from build123d import *

# Parameters (mm, degrees)
SKETCH1_W           = 115
SKETCH1_H           = 45
SKETCH1_R           = 6.125
BOSS_EXTRUDE1_DEPTH = 3
SKETCH2_W           = 5
SKETCH2_H           = 45
BOSS_EXTRUDE2_DEPTH = 5
SKETCH3_R           = 1.45
CUT_EXTRUDE1_DEPTH  = 97.276078541
SKETCH4_W           = 5
SKETCH4_H           = 3
BOSS_EXTRUDE3_DEPTH = 122
BOSS_EXTRUDE5_DEPTH = 3
SKETCH8_W           = 5
SKETCH8_H           = 3
BOSS_EXTRUDE6_DEPTH = 12
SKETCH9_W           = 5
SKETCH9_H           = 3
BOSS_EXTRUDE7_DEPTH = 12
SKETCH10_W          = 5
SKETCH10_H          = 3
SKETCH10_H_2        = 5
BOSS_EXTRUDE8_DEPTH = 41.999995
SKETCH13_R          = 1.5
CUT_EXTRUDE3_DEPTH  = 160.289306921


with BuildPart() as part:
    # Sketch1 → Boss-Extrude1 (new body)
    with BuildSketch(Plane.XY):
        with Locations((-27.46518875, -74.528475384)):
            Rectangle(SKETCH1_W, SKETCH1_H)
        Polygon((-16.746917184, -94.028475384), (-38.183460316, -94.028475384), (-27.46518875, -77.307971742), align=None, mode=Mode.SUBTRACT)
        Polygon((-14.96518875, -57.807971742), (-14.96518875, -91.248979027), (-25.683460316, -74.528475384), align=None, mode=Mode.SUBTRACT)
        Polygon((-38.183460316, -55.028475384), (-16.746917184, -55.028475384), (-27.46518875, -71.748979027), align=None, mode=Mode.SUBTRACT)
        Polygon((-39.96518875, -91.248979027), (-39.96518875, -57.807971742), (-29.246917184, -74.528475384), align=None, mode=Mode.SUBTRACT)
        with BuildLine():
            Line((-11.96518875, -91.907155041), (-11.96518875, -57.149795728))
            Line((-11.96518875, -57.149795728), (0.109576269, -69.224560747))
            ThreePointArc((0.109576269, -69.224560747), (-1.59018875, -74.528475384), (0.109576269, -79.832390022))
            Line((0.109576269, -79.832390022), (-11.96518875, -91.907155041))
        make_face(mode=Mode.SUBTRACT)
        with BuildLine():
            Line((-9.843868406, -55.028475384), (24.913490906, -55.028475384))
            Line((24.913490906, -55.028475384), (12.838725887, -67.103240403))
            ThreePointArc((12.838725887, -67.103240403), (7.53481125, -65.403475384), (2.230896613, -67.103240403))
            Line((2.230896613, -67.103240403), (-9.843868406, -55.028475384))
        make_face(mode=Mode.SUBTRACT)
        with BuildLine():
            Line((27.03481125, -57.149795728), (27.03481125, -91.907155041))
            Line((27.03481125, -91.907155041), (14.960046231, -79.832390022))
            ThreePointArc((14.960046231, -79.832390022), (16.65981125, -74.528475384), (14.960046231, -69.224560747))
            Line((14.960046231, -69.224560747), (27.03481125, -57.149795728))
        make_face(mode=Mode.SUBTRACT)
        with BuildLine():
            Line((12.838725887, -81.953710365), (24.913490906, -94.028475384))
            Line((24.913490906, -94.028475384), (-9.843868406, -94.028475384))
            Line((-9.843868406, -94.028475384), (2.230896613, -81.953710365))
            ThreePointArc((2.230896613, -81.953710365), (7.53481125, -83.653475384), (12.838725887, -81.953710365))
        make_face(mode=Mode.SUBTRACT)
        with BuildLine():
            Line((-81.96518875, -91.907155041), (-81.96518875, -57.149795728))
            Line((-81.96518875, -57.149795728), (-69.890423731, -69.224560747))
            ThreePointArc((-69.890423731, -69.224560747), (-71.59018875, -74.528475384), (-69.890423731, -79.832390022))
            Line((-69.890423731, -79.832390022), (-81.96518875, -91.907155041))
        make_face(mode=Mode.SUBTRACT)
        with BuildLine():
            Line((-79.843868406, -55.028475384), (-45.086509094, -55.028475384))
            Line((-45.086509094, -55.028475384), (-57.161274113, -67.103240403))
            ThreePointArc((-57.161274113, -67.103240403), (-62.46518875, -65.403475384), (-67.769103387, -67.103240403))
            Line((-67.769103387, -67.103240403), (-79.843868406, -55.028475384))
        make_face(mode=Mode.SUBTRACT)
        with BuildLine():
            Line((-42.96518875, -57.149795728), (-42.96518875, -91.907155041))
            Line((-42.96518875, -91.907155041), (-55.039953769, -79.832390022))
            ThreePointArc((-55.039953769, -79.832390022), (-53.34018875, -74.528475384), (-55.039953769, -69.224560747))
            Line((-55.039953769, -69.224560747), (-42.96518875, -57.149795728))
        make_face(mode=Mode.SUBTRACT)
        with BuildLine():
            Line((-45.086509094, -94.028475384), (-79.843868406, -94.028475384))
            Line((-79.843868406, -94.028475384), (-67.769103387, -81.953710365))
            ThreePointArc((-67.769103387, -81.953710365), (-62.46518875, -83.653475384), (-57.161274113, -81.953710365))
            Line((-57.161274113, -81.953710365), (-45.086509094, -94.028475384))
        make_face(mode=Mode.SUBTRACT)
        with Locations((-62.46518875, -74.528475384)):
            Circle(SKETCH1_R, mode=Mode.SUBTRACT)
        with Locations((7.53481125, -74.528475384)):
            Circle(SKETCH1_R, mode=Mode.SUBTRACT)
    boss_extrude1 = extrude(amount=BOSS_EXTRUDE1_DEPTH)

    # Sketch2 → Boss-Extrude2 (add)
    with BuildSketch(Plane(origin=(0, 0, 0), x_dir=(-1, 0, 0), z_dir=(0, 0, -1))):
        with Locations((-27.53481125, -74.528475384)):
            Rectangle(SKETCH2_W, SKETCH2_H)
        with Locations((82.46518875, -74.528475384)):
            Rectangle(SKETCH2_W, SKETCH2_H)
    boss_extrude2 = extrude(amount=BOSS_EXTRUDE2_DEPTH)

    # Sketch3 → Cut-Extrude1 (cut, through all)
    with BuildSketch(Plane(origin=(0, -52.028475384, 0), x_dir=(1, 0, 0), z_dir=(0, 1, 0))):
        with Locations(Location((-82.46518875, 2.5, 0), (0, 0, 180))):
            Circle(SKETCH3_R)
        with Locations(Location((27.53481125, 2.5, 0), (0, 0, 180))):
            Circle(SKETCH3_R)
    cut_extrude1 = extrude(amount=-CUT_EXTRUDE1_DEPTH, mode=Mode.SUBTRACT)

    # Sketch4 → Boss-Extrude3 (add)
    with BuildSketch(Plane(origin=(0, 0, -5), x_dir=(-1, 0, 0), z_dir=(0, 0, -1))):
        with Locations((82.46518875, -95.528475384)):
            Rectangle(SKETCH4_W, SKETCH4_H)
    extrude(amount=BOSS_EXTRUDE3_DEPTH)

    # Mirror3: Boss-Extrude1, Boss-Extrude2, Cut-Extrude1 across plane
    add(boss_extrude1.mirror(Plane(origin=(0, 0, -62), x_dir=(1, 0, 0), z_dir=(0, 0, -1))))
    add(boss_extrude2.mirror(Plane(origin=(0, 0, -62), x_dir=(1, 0, 0), z_dir=(0, 0, -1))))
    add(cut_extrude1.mirror(Plane(origin=(0, 0, -62), x_dir=(1, 0, 0), z_dir=(0, 0, -1))), mode=Mode.SUBTRACT)

    # Sketch7 → Boss-Extrude5 (add)
    with BuildSketch(Plane(origin=(0, -97.028475384, 0), x_dir=(-1, 0, 0), z_dir=(0, -1, 0))):
        Polygon((-30.03481125, 25), (-30.03481125, 17), (-25.03481125, 17), (-25.03481125, 22), (79.96518875, 22), (79.96518875, 17), (84.96518875, 17), (84.96518875, 25), align=None)
        Polygon((79.96518875, 107), (79.96518875, 102), (-25.03481125, 102), (-25.03481125, 107), (-30.03481125, 107), (-30.03481125, 99), (84.96518875, 99), (84.96518875, 107), align=None)
    extrude(amount=-BOSS_EXTRUDE5_DEPTH)

    # Sketch8 → Boss-Extrude6 (add)
    with BuildSketch(Plane.XY.offset(-17)):
        with Locations((27.53481125, -95.528475384)):
            Rectangle(SKETCH8_W, SKETCH8_H)
    extrude(amount=BOSS_EXTRUDE6_DEPTH)

    # Sketch9 → Boss-Extrude7 (add)
    with BuildSketch(Plane(origin=(0, 0, -107), x_dir=(-1, 0, 0), z_dir=(0, 0, -1))):
        with Locations((-27.53481125, -95.528475384)):
            Rectangle(SKETCH9_W, SKETCH9_H)
    extrude(amount=BOSS_EXTRUDE7_DEPTH)

    # Sketch10 → Boss-Extrude8 (add)
    with BuildSketch(Plane(origin=(0, -94.028475384, 0), x_dir=(1, 0, 0), z_dir=(0, 1, 0))):
        with Locations((-82.46518875, 100.5)):
            Rectangle(SKETCH10_W, SKETCH10_H)
        with Locations((-82.46518875, 104.5)):
            Rectangle(SKETCH10_W, SKETCH10_H_2)
        with Locations((-82.46518875, 23.5)):
            Rectangle(SKETCH10_W, SKETCH10_H)
        with Locations((-82.46518875, 19.5)):
            Rectangle(SKETCH10_W, SKETCH10_H_2)
        with Locations((27.53481125, 23.5)):
            Rectangle(SKETCH10_W, SKETCH10_H)
        with Locations((27.53481125, 19.5)):
            Rectangle(SKETCH10_W, SKETCH10_H_2)
        with Locations((27.53481125, 104.5)):
            Rectangle(SKETCH10_W, SKETCH10_H_2)
        with Locations((27.53481125, 100.5)):
            Rectangle(SKETCH10_W, SKETCH10_H)
    extrude(amount=BOSS_EXTRUDE8_DEPTH)

    # Sketch13 → Cut-Extrude3 (cut, through all)
    with BuildSketch(Plane(origin=(0, -52.028475384, 0), x_dir=(1, 0, 0), z_dir=(0, 1, 0))):
        with Locations(Location((27.53481125, 19.5, 0), (0, 0, 270))):
            Circle(SKETCH13_R)
        with Locations(Location((27.53481125, 104.5, 0), (0, 0, 270))):
            Circle(SKETCH13_R)
        with Locations(Location((-82.46518875, 104.5, 0), (0, 0, 270))):
            Circle(SKETCH13_R)
        with Locations(Location((-82.46518875, 19.5, 0), (0, 0, 270))):
            Circle(SKETCH13_R)
    extrude(amount=-CUT_EXTRUDE3_DEPTH, mode=Mode.SUBTRACT)


solid = part.part
The listing builds one solid part. Answer for the finished solid, in the listing's coordinates (mm). A direction names the side the tool comes from. Coordinates: 2 decimals unless noted, no trailing zeros. Order: outer loops, then holes, each group sorted by start corner. A loop starts at its lowest first (then second) coordinate and runs counter-clockwise, first axis right, second up. Notation, with made-up numbers: (-7, 42.25) -> (18, 42.25) arc R17 cw to (18, 57.25) -> close; hole circle Ø1 at (38.25, -20.5). An arc over 180 degrees is marked (long way). Answer in a Markdown table with one row per item. Add a question column.
Item 1: Find section D-D (z = -69.5). Write down the section's boundary in (x, y), then the cut area to 3 significant figures.
Item 2: Find section C-C (x = -35). State how many separate pieces and enclosed holes the cut face has, then the cut area to 3 significant figures.
Item 3: This flat-tipped pin is pushed along its axis until it touches: P1, Ø5.5, axis at x = -83.5, z = -57, coming from the +Y side. Where does it stop, or does it pass through?
Item 4: Find the intervals of material crossed by L1, parallel to X at y = -73, z = -19.5; L2, parallel to X at y = -87.5, z = -105; L3, parallel to Z at x = -63, y = -66, in increasing order. Write a range as from..to.
Item 5: Which of the six approach directions +Z, -Z, +X, -X, +Y, -Y give full straight-line access (tool end or side, diameter ignored) to faces 1 (the face through (25.035, -75, -18)), 2 (the face through (-32.899, -85.785, 1.479)), 3 (the face through (-83, -73, -107))?
Item 6: Determine the mould class of faces 4 (the face through (-51.208, -87.907, -125.479)), 5 (the face through (27, -73, -17)), 6 (the face through (-11.965, -75, 1)), 7 (the face through (27, -52.028, -102)) for opening direction Y: +Y half, -Y half, draft (parallel to the pull), parting line (faces both ways), or undercut.
Item 7: Find section A-A (z = -19.5). Write down the section's boundary in (x, y), then the cut area to 3 significant figures.
Item 8: Find section B-B (z = -2.5). Write down the section's boundary in (x, y), then the cut area to 3 significant figures.
Result set:
| question | item | result |
|---|---|---|
| 1 | outline | (-84.97, -97.03) -> (-79.97, -97.03) -> (-79.97, -94.03) -> (-84.97, -94.03) -> close |
| 1 | area | 15.0 mm² |
| 2 | separate pieces | 10 |
| 2 | enclosed holes | 0 |
| 2 | area | 121 mm² |
| 3 | P1 | stops at y = -94.03 |
| 4 | L1 | x = -84.97..-83.97, -80.97..-79.97, 25.03..26.03, 29.03..30.03 |
| 4 | L2 | x = -84.97..-83.88, -81.05..-79.97, 25.03..26.12, 28.95..30.03 |
| 4 | L3 | z = -127..-124, 0..3 |
| 5 | face 1 | +Y |
| 5 | face 2 | +Z, -Z |
| 5 | face 3 | +X, -X, +Y |
| 6 | face 4 | undercut |
| 6 | face 5 | draft |
| 6 | face 6 | undercut |
| 6 | face 7 | +Y half |
| 7 | outline | (-84.97, -97.03) -> (-83.97, -97.03) -> (-83.97, -52.03) -> (-84.97, -52.03) -> close; (-80.97, -97.03) -> (-79.97, -97.03) -> (-79.97, -52.03) -> (-80.97, -52.03) -> close; (25.03, -97.03) -> (26.03, -97.03) -> (26.03, -52.03) -> (25.03, -52.03) -> close; (29.03, -97.03) -> (30.03, -97.03) -> (30.03, -52.03) -> (29.03, -52.03) -> close |
| 7 | area | 180 mm² |
| 8 | outline | (-84.97, -97.03) -> (-83.92, -97.03) -> (-83.92, -52.03) -> (-84.97, -52.03) -> close; (-81.02, -97.03) -> (-79.97, -97.03) -> (-79.97, -52.03) -> (-81.02, -52.03) -> close; (25.03, -97.03) -> (26.08, -97.03) -> (26.08, -52.03) -> (25.03, -52.03) -> close; (28.98, -97.03) -> (30.03, -97.03) -> (30.03, -52.03) -> (28.98, -52.03) -> close |
| 8 | area | 189 mm² |
